Autodesk Inventor part; units mm, degrees
ref_plane "YZ Plane" through (0, 0, 0) normal (1, 0, 0) x (0, 1, 0)
ref_plane "XZ Plane" through (0, 0, 0) normal (0, 1, 0) x (-1, 0, 0)
ref_plane "XY Plane" through (0, 0, 0) normal (0, 0, 1) x (1, 0, 0)
sketch "Sketch1" plane through (0, 0, 0) normal (0, 0, 1) x (1, 0, 0)
  circle A0 centre (-6.364, 6.364) radius 1
  circle A1 centre (6.364, 6.364) radius 1
  circle A2 centre (6.364, -6.364) radius 1
  circle A3 centre (-6.364, -6.364) radius 1
  line L0 (-12.5, 13.5) -> (12.5, 13.5)
  line L1 (12.5, 13.5) -> (12.5, -13.5)
  line L2 (12.5, -13.5) -> (-12.5, -13.5)
  line L3 (-12.5, -13.5) -> (-12.5, 13.5)
  line L4 (0, 13.5) -> (-9.375, 13.5) construction
  line L5 (0, 6) -> (0, -6) construction
  line L6 (0, 6) -> (0, 6.25) construction
  line L7 (0, -6) -> (0, -6.25) construction
  line L8 (3.9, -6.25) -> (-8.1, -6.25) construction
  line L9 (4.1, 6.25) -> (-8.9, 6.25) construction
  line L10 (0, 6) -> (3.6056, 6) construction
  line L11 (0, 6.25) -> (3.7, 6.25) construction
  line L12 (3.7, 6.25) -> (-3.7, 6.25)
  line L13 (3.7, -6.25) -> (-3.7, -6.25)
  line L14 (0, 0) -> (7.25, 0) construction
  line L15 (0, 0) -> (-7.25, 0)
  arc A4 (-3.7, 6.25) -> (-3.7, -6.25) centre (0.0268, 0) ccw
  arc A5 (3.7, -6.25) -> (3.7, 6.25) centre (-0.0268, 0) ccw
  point P0 (12.5, 0)
  point P1 (0, -6.25)
  dimension "d0" = 27
  dimension "d1" = 25
  dimension "d2" = 9.375
  dimension "d3" = 12
  dimension "d4" = 0.25
  dimension "d5" = 0.25
  dimension "d6" = 3.6056
  dimension "d7" = 3.7
  dimension "d8" = 7.4
  dimension "d10" = 7.4
  dimension "d11" = 7.25
  dimension "d25" = 7.25
extrude "Extrusion1" add sketch "Sketch1" along normal blind 3
sketch "Sketch2" plane through (0, 0, 3) normal (0, 0, 1) x (1, 0, 0)
  line L0 (3.7, -6.25) -> (-3.7, -6.25)
  line L1 (-3.7, 6.25) -> (3.7, 6.25)
  circle A0 centre (-6.364, -6.364) radius 1
  circle A1 centre (6.364, -6.364) radius 1
  circle A2 centre (6.364, 6.364) radius 1
  circle A3 centre (-6.364, 6.364) radius 1
  line L2 (12.5, 13.5) -> (-12.5, 13.5)
  line L3 (-12.5, 13.5) -> (-12.5, -13.5)
  line L4 (-12.5, -13.5) -> (12.5, -13.5)
  line L5 (12.5, -13.5) -> (12.5, 13.5)
  circle A4 centre (0, 0) radius 11
  arc A5 (3.7, -6.25) -> (3.7, 6.25) centre (-0.0268, 0) ccw
  arc A6 (-3.7, 6.25) -> (-3.7, -6.25) centre (0.0268, 0) ccw
  dimension "d14" = 22
extrude "Extrusion2" add sketch "Sketch2" along normal blind 2.5 contours L5 L4 L3 L2
sketch "Sketch3" plane through (-12.5, 13.5, 0) normal (0, 1, 0) x (1, 0, 0)
  line L0 (0, 0) -> (25, 0)
  line L1 (0, 0) -> (0, -5.5)
  line L2 (25, -5.5) -> (0, -5.5)
  line L3 (25, 0) -> (25, -5.5)
  line L4 (12.5, 0) -> (12.5, -5.5) construction
  line L5 (25, -5.5) -> (0, -5.5) construction
  line L6 (12.5, 0) -> (12.5, -2.75) construction
  line L7 (12.5, -2.75) -> (3.125, -2.75) construction
  line L8 (12.5, -2.75) -> (21.875, -2.75) construction
  circle A0 centre (3.125, -2.75) radius 1.4
  circle A1 centre (21.875, -2.75) radius 1.4
  dimension "d17" = 2.75
  dimension "d18" = 9.375
  dimension "d19" = 180
  dimension "d20" = 2.8
  dimension "d21" = 2.8
extrude "Extrusion3" cut sketch "Sketch3" against normal blind 5.5 contours A0 | A1
mirror "Mirror1" about plane through (0, 0, 0) normal (0, 1, 0) of "Extrusion3"
sketch "Sketch4" plane through (0, 0, 5.5) normal (0, 0, 1) x (1, 0, 0)
  circle A0 centre (0, 0) radius 11
  line L0 (12.5, 13.5) -> (-12.5, 13.5)
  line L1 (-12.5, 13.5) -> (-12.5, -13.5)
  line L2 (-12.5, -13.5) -> (12.5, -13.5)
  line L3 (12.5, -13.5) -> (12.5, 13.5)
extrude "Extrusion4" add sketch "Sketch4" along normal blind 1.5
sketch "Sketch5" plane through (0, 0, 7) normal (0, 0, 1) x (1, 0, 0)
  circle A0 centre (0, 0) radius 11.25
  circle A1 centre (0, 0) radius 11
  dimension "d28" = 22.5
extrude "Extrusion5" cut sketch "Sketch5" against normal up to surface (4 mm away)
properties part number "MotorMountv2"
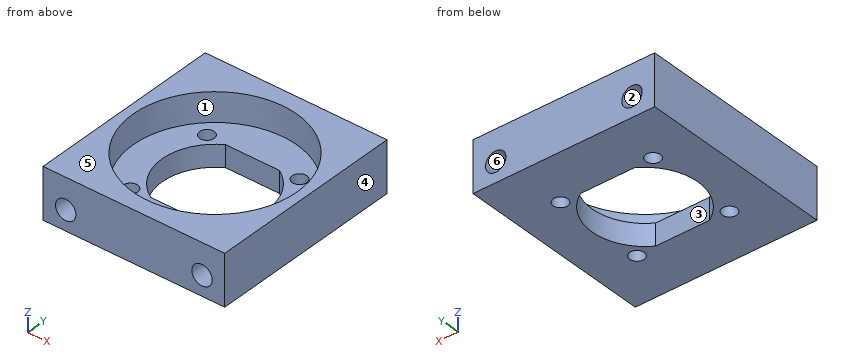
CAD build for the part. Positions are in the model's coordinates, mm. Face numbers are marked on the shaded views. A direction names the side the tool comes from. Give positions to 0.01 mm unless a question says otherwise; leave off trailing zeros. Write each loop counter-clockwise with the first axis right and the second up, starting at its lowest first coordinate (ties: lowest second). Pieces come first, ordered by that corner, then holes. Notation, with made-up numbers: (22, 0.5) - (57, 0.5) arc R16 cw to (57, 16.5) - close; hole circle Ø7 at (-22, 88). An arc over 180 degrees is marked (long way). Put each result on its own line as item: value.
(1) Saw through at D-D (x = 6). List the corners of the cut face in (y, z).
Working result:
outline: (-13.5, 0) - (-7.3, 0) - (-7.3, 3) - (-9.52, 3) - (-9.52, 7) - (-13.5, 7) - close; (-5.43, 0) - (-4.08, 0) - (-4.08, 3) - (-5.43, 3) - close; (4.08, 0) - (5.43, 0) - (5.43, 3) - (4.08, 3) - close; (7.3, 0) - (13.5, 0) - (13.5, 7) - (9.52, 7) - (9.52, 3) - (7.3, 3) - close
(2) Saw through at A-A (y = 0). List the corners of the cut face in (x, z), then the cut area to 3 significant figures.
Working result:
outline: (-12.5, 0) - (-7.25, 0) - (-7.25, 3) - (-11.25, 3) - (-11.25, 7) - (-12.5, 7) - close; (7.25, 0) - (12.5, 0) - (12.5, 7) - (11.25, 7) - (11.25, 3) - (7.25, 3) - close
area: 41.5 mm^2
(3) Pull direction X, two halves, no side cores. Call the marked faces 4, 5 and 6: released by +X, released by -X, zero draft, split by the parting line, or undercut.
Working result:
face 4: released by +X
face 5: zero draft
face 6: undercut
(4) Saw through at B-B (x = 0). List the corners of the cut face in (y, z), then the cut area to 3 significant figures.
Working result:
outline: (-13.5, 0) - (-6.25, 0) - (-6.25, 3) - (-11.25, 3) - (-11.25, 7) - (-13.5, 7) - close; (6.25, 0) - (13.5, 0) - (13.5, 7) - (11.25, 7) - (11.25, 3) - (6.25, 3) - close
area: 61.5 mm^2
(5) Wall check: L1, parallel to X at y = -12.2, z = 2.75 (3 decimals); L2, parallel to Y at x = -3.25, z = 3.75; L3, parallel to X at y = 0, z = 1.5. Give the ranges that are in metal, low to high.
Working result:
L1: -12.5 to -10.775, -7.975 to 7.975, 10.775 to 12.5
L2: -13.5 to -10.77, 10.77 to 13.5
L3: -12.5 to -7.25, 7.25 to 12.5
(6) Tool access for the marked faces 1, 2 and 3: list every direction of +Z, -Z, +X, -X, +Y, -Y with a clear straight run to the whole face (end or side of a thin tool).
Working result:
face 1: +Z
face 2: +Y
face 3: +Z, -Z
(7) Drop flat-ended pins along their axis: pin 1 Ø1.4 at (x, z) = (-9.5, 3) entering from -Y; pin 2 Ø2.5 at (x, y) = (-6.364, 6.364) entering from +Z; pin 3 Ø0.8 at (x, z) = (-8.5, 3) entering from +Y. Give the stop position or say it passes through.
Working result:
pin 1: y = -8
pin 2: z = 3
pin 3: y = 8
(8) Saw through at C-C (z = 3.5). List the corners of the cut face in (x, y), then the cut area to 3 significant figures.
Working result:
outline: (-12.5, -13.5) - (-10.56, -13.5) - (-10.56, -8) - (-8.19, -8) - (-8.19, -13.5) - (8.19, -13.5) - (8.19, -8) - (10.56, -8) - (10.56, -13.5) - (12.5, -13.5) - (12.5, 13.5) - (10.56, 13.5) - (10.56, 8) - (8.19, 8) - (8.19, 13.5) - (-8.19, 13.5) - (-8.19, 8) - (-10.56, 8) - (-10.56, 13.5) - (-12.5, 13.5) - close; hole circle Ø22.5 at (0, 0)
area: 225 mm^2
